For this review, take the finished solid that the model builds, in its own axes (mm). Face numbers are marked on the shaded views. A direction names the side the tool comes from. Round coordinates to 2 decimals unless told otherwise and drop trailing zeros. Loops run counter-clockwise (first coordinate to the right, second up) from the corner with the lowest first, then second, coordinate; pieces in that order, holes last.
1. Clearance check with flat-ended pins moving along their axes: pin 1 Ø5.5 at (x, z) = (6, 14) entering from +Y; pin 2 Ø2 at (x, z) = (-4, 15.5) entering from +Y; pin 3 Ø4.5 at (x, z) = (-4.5, 17.5) entering from -Y; pin 4 Ø6 at (y, z) = (3, 8.5) entering from -X. State where each tip first meets the part, or that it passes through.
2. Consider section A-A on z = 6. State the section outline as (x, y) points.
3. Draft analysis for pull direction Y (two halves, no side actions). For the marked faces 4, 5 and 6, state which applies: released by +Y, released by -Y, zero draft, split by the parting line, or undercut.
4. Consider section B-B on x = 5. State the section outline as (y, z) points, then the cut area to 3 significant figures.
5. To check wall thickness, follow line 1 along Z through (x, y) = (5, 17.2); line 2 along Z through (x, y) = (5, 3.5); line 3 along X through (y, z) = (14.75, 18.5). State the ranges of each line that lie inside material, in increasing order.
6. Consider section C-C on y = 2.5. State the section outline as (x, z) points, then the cut area to 3 significant figures.
7. Consider section D-D on x = -0.25. State the section outline as (y, z) points.
8. Tool access review of the marked faces 1, 2 and 3: name each direction out of +Z, -Z, +X, -X, +Y, -Y from which nothing blocks a thin tool from reaching the whole face with its end or side.
from build123d import *

# Parameters (mm, degrees)
CYLINDER002_R     = 2.6
CYLINDER002_DEPTH = 20
CYLINDER001_R     = 5
CYLINDER001_DEPTH = 16
FILLET_R          = 1
CYLINDER003_R     = 1.6
CYLINDER003_DEPTH = 28
CYLINDER_R        = 2.45
CYLINDER_DEPTH    = 30
BOX001_W          = 10
BOX001_H          = 6
BOX001_DEPTH      = 6
BOX_W             = 12
BOX_H             = 20
BOX_DEPTH         = 20
CHAMFER_SIZE      = 8
CHAMFER001_SIZE   = 3


with BuildPart() as cilindro002:
    # Cylinder002 → Cylinder002 (new body)
    with BuildSketch(Plane(origin=(-9, 10, 6), x_dir=(0, 0, -1), z_dir=(1, 0, 0))):
        Circle(CYLINDER002_R)
    extrude(amount=CYLINDER002_DEPTH)


with BuildPart() as fillet_body:
    # Cylinder001 → Cylinder001 (new body)
    with BuildSketch(Plane(origin=(6, 10, 6), x_dir=(0, 0, -1), z_dir=(1, 0, 0))):
        Circle(CYLINDER001_R)
    extrude(amount=CYLINDER001_DEPTH)

    # Fillet
    fillet_edges = [fillet_body.edges().sort_by_distance(p)[0] for p in [
        (6, 10, 11),
    ]]
    fillet(fillet_edges, radius=FILLET_R)


with BuildPart() as fillet_body_1:
    # Fillet placement: moved
    add(fillet_body.part.moved(Location((-4, 0, 0))))


with BuildPart() as cilindro003:
    # Cylinder003 → Cylinder003 (new body)
    with BuildSketch(Plane(origin=(7, 23, 15), x_dir=(1, 0, 0), z_dir=(0, -1, 0))):
        Circle(CYLINDER003_R)
    extrude(amount=CYLINDER003_DEPTH)


with BuildPart() as cilindro:
    # Cylinder → Cylinder (new body)
    with BuildSketch(Plane(origin=(7, 44, 15), x_dir=(1, 0, 0), z_dir=(0, -1, 0))):
        Circle(CYLINDER_R)
    extrude(amount=CYLINDER_DEPTH)


with BuildPart() as cubo001:
    # Box001 → Box001 (new body)
    with BuildSketch(Plane(origin=(-4, 7, 14), x_dir=(1, 0, 0), z_dir=(0, 0, 1))):
        with Locations((5, 3)):
            Rectangle(BOX001_W, BOX001_H)
    extrude(amount=BOX001_DEPTH)


with BuildPart() as chamfer001:
    # Box → Box (new body)
    with BuildSketch(Plane.XY):
        with Locations((6, 10)):
            Rectangle(BOX_W, BOX_H)
    extrude(amount=BOX_DEPTH)

    # Fusion: union Cubo001
    add(cubo001.part)

    # Cut: cut Cilindro
    add(cilindro.part, mode=Mode.SUBTRACT)

    # Cut001: cut Cilindro003
    add(cilindro003.part, mode=Mode.SUBTRACT)

    # Chamfer
    chamfer_edges = [chamfer001.edges().sort_by_distance(p)[0] for p in [
        (12, 10, 0),
    ]]
    chamfer(chamfer_edges, length=CHAMFER_SIZE)


with BuildPart() as chamfer001_1:
    # Chamfer placement: moved
    add(chamfer001.part.moved(Location((-2, 0, 0))))

    # Cut002: cut Fillet body
    add(fillet_body_1.part, mode=Mode.SUBTRACT)

    # Cut003: cut Cilindro002
    add(cilindro002.part, mode=Mode.SUBTRACT)

    # Chamfer001
    chamfer001_edges = [chamfer001_1.edges().sort_by_distance(p)[0] for p in [
        (10, 0, 14),
    ]]
    chamfer(chamfer001_edges, length=CHAMFER001_SIZE)


solid = chamfer001_1.part
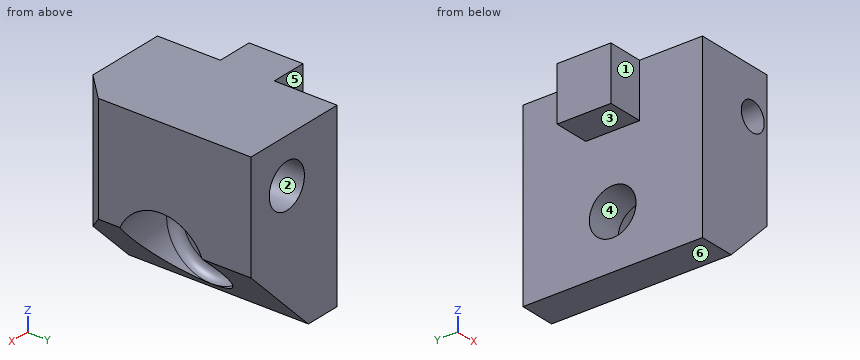
Resolved:
1. pin 1: stops at y = 20
1. pin 2: stops at y = 13
1. pin 3: stops at y = 7
1. pin 4: stops at x = -2
2. outline: (-2, 0) - (7, 0) - (8, 1) - (8, 5) - (3, 5) arc R1 cw to (2, 6) - (2, 7.4) - (-2, 7.4) - close; (-2, 12.6) - (2, 12.6) - (2, 14) arc R1 cw to (3, 15) - (8, 15) - (8, 20) - (-2, 20) - close
3. face 4: undercut
3. face 5: released by +Y
3. face 6: zero draft
4. outline: (0, 3) - (6, 3) arc R5 cw (long way) to (14, 3) - (20, 3) - (20, 12.55) - (14, 12.55) - (14, 13.4) - (0, 13.4) - close; (0, 16.6) - (14, 16.6) - (14, 17.45) - (20, 17.45) - (20, 20) - (0, 20) - close
4. area: 198 mm2
5. line 1: z = 3 to 12.55, 17.45 to 20
5. line 2: z = 3 to 13.4, 16.6 to 20
5. line 3: x = -2 to 10
6. outline: (-2, 0) - (2, 0) - (9.5, 7.5) - (9.5, 20) - (-2, 20) - close; hole circle Ø3.2 at (5, 15)
6. area: 194 mm2
7. outline: (0, 0) - (20, 0) - (20, 20) - (0, 20) - close; hole circle Ø5.2 at (10, 6)
8. face 1: +Z, -Z, -X, -Y
8. face 2: +Y
8. face 3: -Z, -X, +Y, -Y
